```python
from build123d import *

# Parameters (mm, degrees)
SALIENTE_EXTRUIR1_DEPTH = 1.5
CROQUIS2_W              = 30
CROQUIS2_H              = 30
CORTAR_EXTRUIR1_DEPTH   = 123.41919068


with BuildPart() as part:
    # Croquis1 → Saliente-Extruir1 (new body)
    with BuildSketch(Plane(origin=(0, 0, 0), x_dir=(1, 0, 0), z_dir=(0, 1, 0))):
        with BuildLine():
            Line((-10.354497354, 18.78659612), (-10.354497354, -55.21340388))
            Line((-10.354497354, -55.21340388), (-10.354497354, -102.21340388))
            Line((-10.354497354, -102.21340388), (9.645502646, -102.21340388))
            Line((9.645502646, -102.21340388), (9.645502646, -55.21340388))
            Line((9.645502646, -55.21340388), (9.645502646, 18.78659612))
            ThreePointArc((9.645502646, 18.78659612), (-0.354497354, 19.704716991), (-10.354497354, 18.78659612))
        make_face()
        with BuildLine():
            ThreePointArc((53.645502646, -25.21340388), (38.478478323, 3.619571798), (9.645502646, 18.78659612))
            Line((9.645502646, 18.78659612), (9.645502646, -55.21340388))
            Line((9.645502646, -55.21340388), (39.645502646, -55.21340388))
            Line((39.645502646, -55.21340388), (39.645502646, -54.71340388))
            ThreePointArc((39.645502646, -54.71340388), (42.427988224, -47.995889459), (49.145502646, -45.21340388))
            Line((49.145502646, -45.21340388), (66.645502646, -45.21340388))
            Line((66.645502646, -45.21340388), (66.645502646, -25.21340388))
            Line((66.645502646, -25.21340388), (53.645502646, -25.21340388))
        make_face()
        with BuildLine():
            Line((-40.354497354, -54.71340388), (-40.354497354, -55.21340388))
            Line((-40.354497354, -55.21340388), (-10.354497354, -55.21340388))
            Line((-10.354497354, -55.21340388), (-10.354497354, 18.78659612))
            ThreePointArc((-10.354497354, 18.78659612), (-39.187473032, 3.619571798), (-54.354497354, -25.21340388))
            Line((-54.354497354, -25.21340388), (-67.354497354, -25.21340388))
            Line((-67.354497354, -25.21340388), (-67.354497354, -45.21340388))
            Line((-67.354497354, -45.21340388), (-49.854497354, -45.21340388))
            ThreePointArc((-49.854497354, -45.21340388), (-43.136982933, -47.995889459), (-40.354497354, -54.71340388))
        make_face()
        with BuildLine():
            Line((-10.354497354, 31.78659612), (-10.354497354, 18.78659612))
            ThreePointArc((-10.354497354, 18.78659612), (-0.354497354, 19.704716991), (9.645502646, 18.78659612))
            Line((9.645502646, 18.78659612), (9.645502646, 31.78659612))
            Line((9.645502646, 31.78659612), (-10.354497354, 31.78659612))
        make_face()
    extrude(amount=SALIENTE_EXTRUIR1_DEPTH)

    # Croquis2 → Cortar-Extruir1 (cut, through all)
    with BuildSketch(Plane(origin=(0, 1.5, 0), x_dir=(1, 0, 0), z_dir=(0, 1, 0))):
        with Locations((-17.354497354, -28.01340388)):
            Rectangle(CROQUIS2_W, CROQUIS2_H)
    extrude(amount=-CORTAR_EXTRUIR1_DEPTH, mode=Mode.SUBTRACT)


solid = part.part
```
Check sheet for the modelled part. Datum: model origin and axes. Units: mm. Give positions to 0.01 mm unless a question says otherwise; leave off trailing zeros. Loops run counter-clockwise (first coordinate to the right, second up) from the corner with the lowest first, then second, coordinate; pieces in that order, holes last. Notation, with made-up numbers: M 8,29.5 L 20,29.5 A26 cw 20,59.5 Z; hole C 79.25,-29.5 d1. An arc over 180 degrees is marked long. Answer in a Markdown table with one row per item.
1) Cross-section at C-C (z = 15). Enter the section's corners in (x, y).
Solutions:
| item | result |
|---|---|
| outline | M -51.42,0 L -32.35,0 L -32.35,1.5 L -51.42,1.5 Z; M -2.35,0 L 50.71,0 L 50.71,1.5 L -2.35,1.5 Z |
2) Thickness scan on line 1 (Z direction, x = -6.5, y = 1.2); line 2 (X direction, y = 0.1, z = 28.5); line 3 (X direction, y = 0.7, z = 82). Record the ranges inside material, lowest first.
Solutions:
| item | result |
|---|---|
| line 1 | z = -31.79 to 13.01, 43.01 to 102.21 |
| line 2 | x = -67.35 to -32.35, -2.35 to 66.65 |
| line 3 | x = -10.35 to 9.65 |
3) Cross-section at B-B (x = -8). Enter the section's corners in (y, z), plus the area to 3 significant figures.
Solutions:
| item | result |
|---|---|
| outline | M 0,-31.79 L 1.5,-31.79 L 1.5,13.01 L 0,13.01 Z; M 0,43.01 L 1.5,43.01 L 1.5,102.21 L 0,102.21 Z |
| area | 156 mm^2 |
4) Cross-section at D-D (x = 56). Enter the section's corners in (y, z), plus the area to 3 significant figures.
Solutions:
| item | result |
|---|---|
| outline | M 0,25.21 L 1.5,25.21 L 1.5,45.21 L 0,45.21 Z |
| area | 30.0 mm^2 |
5) Depth check by flat-ended pin: pin 1 (0.8 mm diameter, centred on y = 0.5, z = 24, fed in from -X); pin 2 (0.8 mm diameter, centred on x = -14, y = 1, fed in from +Z); pin 3 (10 mm diameter, centred on x = 48, z = 33.5, fed in from -Y); pin 4 (0.8 mm diameter, centred on y = 1, z = 71, fed in from -X). Enter the tip coordinate at first touch or a pass-through.
Solutions:
| item | result |
|---|---|
| pin 1 | stops at x = -54.2 |
| pin 2 | stops at z = 55.21 |
| pin 3 | stops at y = 0 |
| pin 4 | stops at x = -10.35 |
6) Cross-section at A-A (y = 0.85). Enter the section's corners in (x, z), plus the area to 3 significant figures.
Solutions:
| item | result |
|---|---|
| outline | M -67.35,25.21 L -54.35,25.21 A54.92 ccw -10.35,-18.79 L -10.35,-31.79 L 9.65,-31.79 L 9.65,-18.79 A54.92 ccw 53.65,25.21 L 66.65,25.21 L 66.65,45.21 L 49.15,45.21 A9.5 cw 39.65,54.71 L 39.65,55.21 L 9.65,55.21 L 9.65,102.21 L -10.35,102.21 L -10.35,55.21 L -40.35,55.21 L -40.35,54.71 A9.5 cw -49.85,45.21 L -67.35,45.21 Z; hole M -32.35,13.01 L -2.35,13.01 L -2.35,43.01 L -32.35,43.01 Z |
| area | 7,450 mm^2 |
